from build123d import *

# Parameters (mm, degrees)
EXTRUDE_1_DEPTH = 40
SKETCH_3_W      = 1.92
SKETCH_3_H      = 1.335454545
EXTRUDE_2_DEPTH = 40
SKETCH_4_W      = 1.92
SKETCH_4_H      = 40
EXTRUDE_3_DEPTH = 1
SKETCH_5_W      = 1.92
SKETCH_5_H      = 40
EXTRUDE_4_DEPTH = 10
SKETCH_7_W      = 10
SKETCH_7_H      = 2
EXTRUDE_5_DEPTH = 40


with BuildPart() as part:
    # 草圖2 → 填料-伸長1 (new body)
    with BuildSketch(Plane(origin=(0, 0, 0), x_dir=(1, 0, 0), z_dir=(0, 1, 0))):
        Polygon((-1.169090909, -3.013636364), (-1.169090909, -1.559090909), (-2.659090909, -1.559090909), (-2.659090909, 3.340909091), (2.240909091, 3.340909091), (2.240909091, -1.559090909), (0.750909091, -1.559090909), (0.750909091, -3.013636364), align=None)
    extrude(amount=EXTRUDE_1_DEPTH)

    # 草圖3 → 填料-伸長2 (add)
    with BuildSketch(Plane(origin=(0, 40, 0), x_dir=(1, 0, 0), z_dir=(0, 1, 0))):
        with Locations((-0.209090909, -3.681363637)):
            Rectangle(SKETCH_3_W, SKETCH_3_H)
    extrude(amount=-EXTRUDE_2_DEPTH)

    # 草圖4 → 填料-伸長3 (add)
    with BuildSketch(Plane.XY.offset(4.349090909)):
        with Locations((-0.209090909, 20)):
            Rectangle(SKETCH_4_W, SKETCH_4_H)
    extrude(amount=EXTRUDE_3_DEPTH)

    # 草圖5 → 填料-伸長4 (add)
    with BuildSketch(Plane.XY.offset(5.349090909)):
        with Locations((-0.209090909, 20)):
            Rectangle(SKETCH_5_W, SKETCH_5_H)
    extrude(amount=EXTRUDE_4_DEPTH)

    # 草圖7 → 填料-伸長5 (add)
    with BuildSketch(Plane(origin=(0, 40, 0), x_dir=(1, 0, 0), z_dir=(0, 1, 0))):
        with Locations((-0.209090909, -14.349090909)):
            Rectangle(SKETCH_7_W, SKETCH_7_H)
    extrude(amount=-EXTRUDE_5_DEPTH)


solid = part.part
Part model, mm, in its own coordinate system. A direction names the side the tool comes from. Round coordinates to 2 decimals unless told otherwise and drop trailing zeros. Write each loop counter-clockwise with the first axis right and the second up, starting at its lowest first coordinate (ties: lowest second). Pieces come first, ordered by that corner, then holes. Notation, with made-up numbers: (81, 55.5) - (128, 55.5) arc R15 ccw to (128, 61.5) - close; hole circle Ø2 at (28, 56.25). An arc over 180 degrees is marked (long way). Use CSV: the item, a comma, the result in double quotes.
Item 1: Pull direction Z, two halves, no side cores. Call faces 1 (the flat face through (-1.169, 20, 7)), 2 (the flat face through (0, 20, 15.349)), 3 (the flat face through (2.241, 20, -1)): pulls with the +Z half, pulls with the -Z half, needs draft (parallel to the pull), parting line crosses it, or undercut.
Results list:
face 1,"undercut"
face 2,"pulls with the +Z half"
face 3,"needs draft"
Item 2: Wall check: L1, parallel to Z at x = -2.5, y = 24.5; L2, parallel to X at y = 24.5, z = 7; L3, parallel to X at y = 5, z = 1. Give the ranges that are in metal, low to high.
Results list:
L1,"z = -3.34 to 1.56, 13.35 to 15.35"
L2,"x = -1.17 to 0.75"
L3,"x = -2.66 to 2.24"
Item 3: Tool access for faces 4 (the flat face through (-2, 20, 1.559)), 5 (the flat face through (3, 20, 13.349)), 6 (the flat face through (-2.659, 20, -1)), 7 (the flat face through (-1, 40, 7)): list every direction of +Z, -Z, +X, -X, +Y, -Y with a clear straight run to the whole face (end or side of a thin tool).
Results list:
face 4,"-X, +Y, -Y"
face 5,"+X, +Y, -Y"
face 6,"-Z, -X, +Y, -Y"
face 7,"+Z, -Z, +X, -X, +Y"
Item 4: Slice it at B-B, the plane z = -1. Write the cut outline in (x, y), then the cut area to 3 significant figures.
Results list:
outline,"(-2.66, 0) - (2.24, 0) - (2.24, 40) - (-2.66, 40) - close"
area,"196 mm²"
Item 5: Flat gauge pins, fed straight in: P1, Ø1.5, axis at y = 23.5, z = 0, coming from the -X side; P2, Ø6, axis at y = 12, z = 6, coming from the +X side; P3, Ø1.5, axis at y = 23, z = -1.5, coming from the +X side. Where does each tip first touch, or does it go through?
Results list:
P1,"stops at x = -2.66"
P2,"stops at x = 0.75"
P3,"stops at x = 2.24"
Item 6: Slice it at C-C, the plane x = -4.5. Write the cut outline in (y, z).
Results list:
outline,"(0, 13.35) - (40, 13.35) - (40, 15.35) - (0, 15.35) - close"
Item 7: Slice it at A-A, the plane y = 5. Write the cut outline in (x, z).
Results list:
outline,"(-5.21, 13.35) - (-1.17, 13.35) - (-1.17, 1.56) - (-2.66, 1.56) - (-2.66, -3.34) - (2.24, -3.34) - (2.24, 1.56) - (0.75, 1.56) - (0.75, 13.35) - (4.79, 13.35) - (4.79, 15.35) - (-5.21, 15.35) - close"
